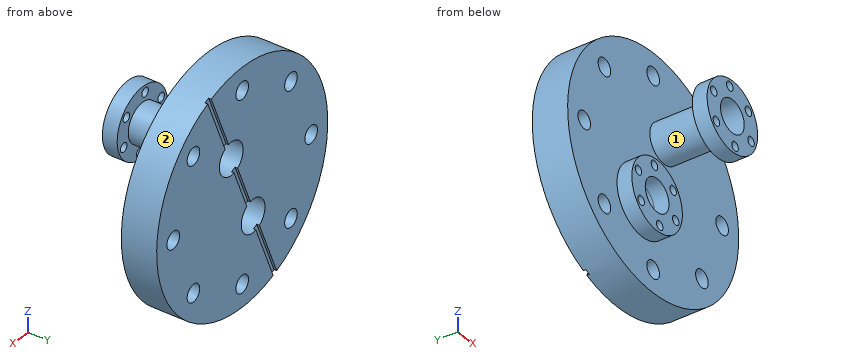
```python
from build123d import *

# Parameters (mm, degrees)
SKETCH1_R         = 57.15
EXTRUDE1_DEPTH    = 17.272
SKETCH3_R         = 4.2164
EXTRUDE2_DEPTH    = 83.647244261
CIRPATTERN1_COUNT = 8
SKETCH5_R         = 9.4996
SKETCH5_R_2       = 7.9375
EXTRUDE3_DEPTH    = 33.3375
EXTRUDE4_START    = -7.239
SKETCH6_R         = 16.891
SKETCH6_R_2       = 7.9375
EXTRUDE4_DEPTH    = 7.239
EXTRUDE5_REACH    = 97.36
SKETCH7_R         = 2.1844
CIRPATTERN2_COUNT = 6
SKETCH8_R         = 7.9375
EXTRUDE6_DEPTH    = 96.360193426
SKETCH9_R         = 16.891
SKETCH9_R_2       = 7.9375
EXTRUDE7_DEPTH    = 7.239
SKETCH11_R        = 7.9375
EXTRUDE8_DEPTH    = 85.931600139
SKETCH12_R        = 2.1844
EXTRUDE9_DEPTH    = 7.239
CIRPATTERN3_COUNT = 6
EXTRUDE10_DEPTH   = 1.27


with BuildPart() as part:
    # Sketch1 → Extrude1 (new body)
    with BuildSketch(Plane(origin=(0, 0, 0), x_dir=(1, 0, 0), z_dir=(0, 1, 0))):
        with Locations(Location((0, 0, 0), (0, 0, 270))):
            Circle(SKETCH1_R)
    extrude(amount=EXTRUDE1_DEPTH)

    # Sketch3 → Extrude2 (cut, through all)
    with BuildSketch(Plane.XZ):
        with Locations(Location((0, 46.0756, 0), (0, 0, 270))):
            Circle(SKETCH3_R)
    extrude2 = extrude(amount=-EXTRUDE2_DEPTH, mode=Mode.SUBTRACT)

    # CirPattern1: Extrude2 ×8 about axis
    cirpattern1_axis = Axis((0, 0, 0), (0, 1, 0))
    for i in range(1, CIRPATTERN1_COUNT):
        add(extrude2.rotate(cirpattern1_axis, i * 360 / CIRPATTERN1_COUNT), mode=Mode.SUBTRACT)

    # Sketch5 → Extrude3 (add)
    with BuildSketch(Plane.XZ):
        with Locations(Location((7.290119387, 17.599905094, 0), (0, 0, 90))):
            Circle(SKETCH5_R)
        with Locations(Location((7.290119387, 17.599905094, 0), (0, 0, 270))):
            Circle(SKETCH5_R_2, mode=Mode.SUBTRACT)
    extrude(amount=EXTRUDE3_DEPTH)

    # Sketch6 → Extrude4 (add)
    with BuildSketch(Plane.XZ.offset(33.3375).offset(EXTRUDE4_START)):
        with Locations(Location((7.290119387, 17.599905094, 0), (0, 0, 270))):
            Circle(SKETCH6_R)
        with Locations(Location((7.290119387, 17.599905094, 0), (0, 0, 270))):
            Circle(SKETCH6_R_2, mode=Mode.SUBTRACT)
    extrude(amount=EXTRUDE4_DEPTH)

    # Sketch7 → Extrude5 (cut, up to next)
    with BuildSketch(Plane.XZ.offset(33.3375), mode=Mode.PRIVATE) as extrude5_sk1:
        with Locations(Location((-3.410154455, 9.389296197, 0), (0, 0, 270))):
            Circle(SKETCH7_R)
    extrude5_tool1 = extrude(extrude5_sk1.sketch, amount=-EXTRUDE5_REACH, mode=Mode.PRIVATE) & part.part
    extrude5 = extrude5_tool1.solids().sort_by_distance((-3.410154, -33.3375, 9.389296))[0]
    add(extrude5, mode=Mode.SUBTRACT)

    # CirPattern2: Extrude5 ×6 about axis
    cirpattern2_axis = Axis((7.290119387, 0, 17.599905094), (0, 1, 0))
    for i in range(1, CIRPATTERN2_COUNT):
        add(extrude5.rotate(cirpattern2_axis, i * 360 / CIRPATTERN2_COUNT), mode=Mode.SUBTRACT)

    # Sketch8 → Extrude6 (cut, through all)
    with BuildSketch(Plane.XZ.offset(33.3375)):
        with Locations(Location((7.290119387, 17.599905094, 0), (0, 0, 270))):
            Circle(SKETCH8_R)
    extrude(amount=-EXTRUDE6_DEPTH, mode=Mode.SUBTRACT)

    # Sketch9 → Extrude7 (add)
    with BuildSketch(Plane.XZ):
        with Locations(Location((-7.290119387, -17.599905094, 0), (0, 0, 90))):
            Circle(SKETCH9_R)
        with Locations(Location((-7.290119387, -17.599905094, 0), (0, 0, 270))):
            Circle(SKETCH9_R_2, mode=Mode.SUBTRACT)
    extrude(amount=EXTRUDE7_DEPTH)

    # Sketch11 → Extrude8 (cut, through all)
    with BuildSketch(Plane.XZ.offset(7.239)):
        with Locations(Location((-7.290119387, -17.599905094, 0), (0, 0, 270))):
            Circle(SKETCH11_R)
    extrude(amount=-EXTRUDE8_DEPTH, mode=Mode.SUBTRACT)

    # Sketch12 → Extrude9 (cut)
    with BuildSketch(Plane.XZ.offset(7.239)):
        with Locations(Location((3.410154455, -9.389296197, 0), (0, 0, 270))):
            Circle(SKETCH12_R)
    extrude9 = extrude(amount=-EXTRUDE9_DEPTH, mode=Mode.SUBTRACT)

    # CirPattern3: Extrude9 ×6 about axis
    cirpattern3_axis = Axis((-7.290119387, 0, -17.599905094), (0, 1, 0))
    for i in range(1, CIRPATTERN3_COUNT):
        add(extrude9.rotate(cirpattern3_axis, i * 360 / CIRPATTERN3_COUNT), mode=Mode.SUBTRACT)

    # Sketch13 → Extrude10 (cut)
    with BuildSketch(Plane(origin=(0, 17.272, 0), x_dir=(1, 0, 0), z_dir=(0, 1, 0))):
        Polygon((-24.155973891, 61.636349712), (-26.502627904, 60.664333794), (25.660622812, -65.268893542), (28.007276825, -64.296877624), align=None)
    extrude(amount=-EXTRUDE10_DEPTH, mode=Mode.SUBTRACT)


solid = part.part
```
The listing builds one solid part. Answer for the finished solid, in the listing's coordinates (mm). Face numbers are marked on the shaded views. A direction names the side the tool comes from. Give positions to 0.01 mm unless a question says otherwise; leave off trailing zeros. Loops run counter-clockwise (first coordinate to the right, second up) from the corner with the lowest first, then second, coordinate; pieces in that order, holes last. Notation, with made-up numbers: M 32.5,-3 L 78.5,-3 A17 cw 78.5,11 Z; hole C 59.5,-14.75 d11. An arc over 180 degrees is marked long. One line per item, written item: value.
1. Section D-D on y = -11 is taken. Determine the outline of the cut face in (x, z) (1 decimal).
Found:
outline: C 7.3,17.6 d19; hole C 7.3,17.6 d15.9
2. Section B-B on z = 48 is taken. Determine the outline of the cut face in (x, y).
Found:
outline: M -31.02,0 L -3.75,0 L -3.75,17.27 L -31.02,17.27 Z; M 3.75,0 L 31.02,0 L 31.02,17.27 L 21.26,17.27 L 21.26,16 L 18.51,16 L 18.51,17.27 L 3.75,17.27 Z
3. Find the intervals of material crossed by probe 1 along X at (y, z) = (3, -47.5); probe 2 along Y at (x, z) = (-50.5, -6); probe 3 along Z at (x, y) = (1, -15.5), in increasing order.
Found:
probe 1: -31.78 to -3.97, 3.97 to 31.78
probe 2: 0 to 17.27
probe 3: 10.48 to 12.76, 22.44 to 24.72
4. Section A-A on y = -2 is taken. State how many separate pieces and enclosed holes the cut face has, plus the area to 3 significant figures.
Found:
separate pieces: 2
enclosed holes: 8
area: 694 mm^2
5. Each of these flat-tipped pins is pushed along its axis until it touches: P1, Ø4, axis at x = -9.05, z = -4.23, coming from the -Y side; P2, Ø5, axis at y = -9, z = 6.5, coming from the -X side; P3, Ø2, axis at x = -9, y = 8.5, coming from the +Z side. Where does it stop, or does it pass through?
Found:
P1: y = 0
P2: x = 3.25
P3: z = 56.59
6. For the marked faces 1 and 2, determine the directions among +Z, -Z, +X, -X, +Y, -Y from which every point of the face is accessible in a straight line to the end or side of a thin tool.
Found:
face 1: none
face 2: +Y, -Y
